Verification items for the finished model (mm, model axes). Coordinates: 2 decimals unless noted, no trailing zeros. Order: outer loops, then holes, each group sorted by start corner. A loop starts at its lowest first (then second) coordinate and runs counter-clockwise, first axis right, second up. Notation, with made-up numbers: (89.25, 77.25) -> (130.25, 77.25) arc R9 ccw to (130.25, 89.25) -> close; hole circle Ø7 at (42.5, 85.25). An arc over 180 degrees is marked (long way). Use CSV: the item, a comma, the result in double quotes. Start each with the question number.
1) Sectioned sample at B-B on y = -209. Record the boundary of the cut face in (x, z) (3 decimals).
2) Scan lines: line 1 along Z through (x, y) = (0.5, -213) (3 decimals); line 2 along Z through (x, y) = (9.2, -41.91) (3 decimals). Record each from-to range of solid material in increasing order.
3) Sectioned sample at A-A on x = -1. Record the boundary of the cut face in (y, z) (3 decimals).
4) Sectioned sample at C-C on y = -48.5. Record the boundary of the cut face in (x, z) (3 decimals), then the cut area to 3 significant figures.
5) Go/stop test with flat-tipped pins: pin 1 (2.5 mm diameter, centred on y = -41.91, z = -4.318, fed in from +X) (1 decimal); pin 2 (0.5 mm diameter, centred on x = 1, z = -9, fed in from +Y). Record where each tip stops, or that it passes through.
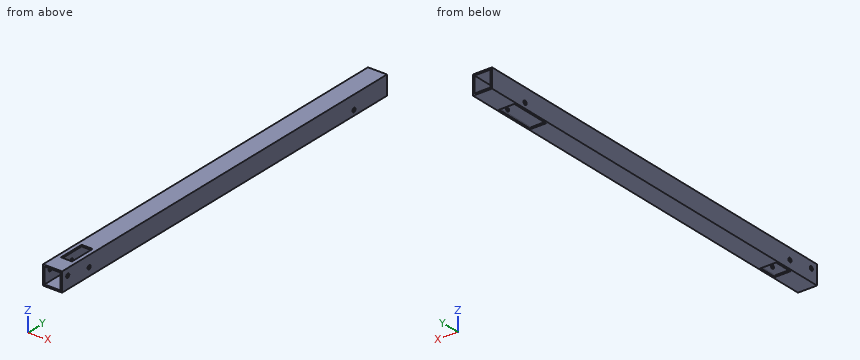
from build123d import *

# Parameters (mm, degrees)
F0_W          = 19.05
F0_H          = 19.05
F0_W_2        = 16.002
F0_H_2        = 16.002
F1_DEPTH      = 412.75
F2_R          = 1.9812
F3_DEPTH      = 25.4
F3_DEPTH_BACK = 25.4
F4_W          = 15.24
F4_H          = 40.386
F4_H_2        = 18.415
F5_DEPTH      = 6.35
F6_W          = 11.049
F6_H          = 26.162
F7_DEPTH      = 6.35


with BuildPart() as f1:
    # F0 (on Front) → F1 (new body)
    with BuildSketch(Plane.XZ):
        Rectangle(F0_W, F0_H)
        Rectangle(F0_W_2, F0_H_2, mode=Mode.SUBTRACT)
    extrude(amount=F1_DEPTH)

    # F2 (on Right) → F3 (cut, two sides)
    with BuildSketch(Plane.YZ) as f3_sk:
        with Locations((-405.511, 2.667)):
            Circle(F2_R)
        with Locations((-378.333, -1.397)):
            Circle(F2_R)
        with Locations((-41.91, -4.318)):
            Circle(F2_R)
    extrude(amount=-F3_DEPTH, mode=Mode.SUBTRACT)
    extrude(f3_sk.sketch, amount=F3_DEPTH_BACK, mode=Mode.SUBTRACT)

    # F4 (on face) → F5 (cut)
    with BuildSketch(Plane(origin=(0, 0, -9.525), x_dir=(1, 0, 0), z_dir=(0, 0, -1))):
        with Locations((0, 50.927)):
            Rectangle(F4_W, F4_H)
        with Locations((0, 372.1735)):
            Rectangle(F4_W, F4_H_2)
    extrude(amount=-F5_DEPTH, mode=Mode.SUBTRACT)

    # F6 (on face) → F7 (cut)
    with BuildSketch(Plane.XY.offset(9.525)):
        with Locations((0, -381.889)):
            Rectangle(F6_W, F6_H)
    extrude(amount=-F7_DEPTH, mode=Mode.SUBTRACT)


solid = f1.part
Answers follow:
1,outline,"(-9.525, -9.525) -> (9.525, -9.525) -> (9.525, 9.525) -> (-9.525, 9.525) -> close; hole (-8.001, -8.001) -> (8.001, -8.001) -> (8.001, 8.001) -> (-8.001, 8.001) -> close"
2,line 1,"z = -9.525 to -8.001, 8.001 to 9.525"
2,line 2,"z = -9.525 to -6.299, -2.337 to 9.525"
3,outline,"(-412.75, -9.525) -> (-381.381, -9.525) -> (-381.381, -8.001) -> (-412.75, -8.001) -> close; (-412.75, 8.001) -> (-394.97, 8.001) -> (-394.97, 9.525) -> (-412.75, 9.525) -> close; (-368.808, 8.001) -> (0, 8.001) -> (0, 9.525) -> (-368.808, 9.525) -> close; (-362.966, -9.525) -> (-71.12, -9.525) -> (-71.12, -8.001) -> (-362.966, -8.001) -> close; (-30.734, -9.525) -> (0, -9.525) -> (0, -8.001) -> (-30.734, -8.001) -> close"
4,outline,"(-9.525, -9.525) -> (-7.62, -9.525) -> (-7.62, -8.001) -> (-8.001, -8.001) -> (-8.001, 8.001) -> (8.001, 8.001) -> (8.001, -8.001) -> (7.62, -8.001) -> (7.62, -9.525) -> (9.525, -9.525) -> (9.525, 9.525) -> (-9.525, 9.525) -> close"
4,area,"83.6 mm²"
5,pin 1,"passes through"
5,pin 2,"stops at y = 0"
